Geometry check sheet. Reference: the model listing, model coordinates, mm. Round coordinates to 2 decimals unless told otherwise and drop trailing zeros. Loops run counter-clockwise (first coordinate to the right, second up) from the corner with the lowest first, then second, coordinate; pieces in that order, holes last. Notation, with made-up numbers: (4, -17) - (12, -17) arc R15 cw to (12, 4) - close; hole circle Ø2 at (-31, -34). An arc over 180 degrees is marked (long way). Write item = value, one per line.
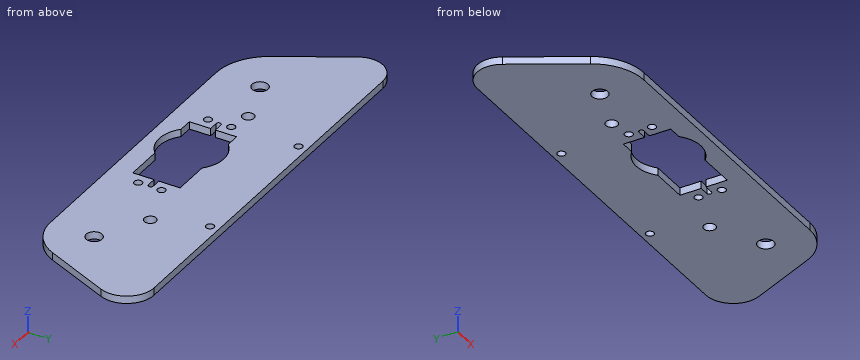
```python
from build123d import *

# Parameters (mm, degrees)
SKETCH1_R           = 3.429
SKETCH1_R_2         = 2.54
BOSS_EXTRUDE1_DEPTH = 3.2004
SKETCH2_R           = 1.7272
CUT_EXTRUDE1_DEPTH  = 3.2004
SKETCH5_R           = 1.7272
SKETCH5_W           = 40.894
SKETCH5_H           = 20.32
CUT_EXTRUDE3_DEPTH  = 4.2004
CUT_EXTRUDE4_DEPTH  = 3.2004
SKETCH9_R           = 13.885201093
CUT_EXTRUDE7_DEPTH  = 3.2004


with BuildPart() as part:
    # Sketch1 → Boss-Extrude1 (new body)
    with BuildSketch(Plane.XY):
        with BuildLine():
            Line((0, 0), (120.015, 0))
            ThreePointArc((120.015, 0), (130.351788397, 3.075697789), (137.325636158, 11.302152593))
            Line((137.325636158, 11.302152593), (149.69326877, 39.451329485))
            ThreePointArc((149.69326877, 39.451329485), (148.774539583, 50.600046625), (138.937102863, 55.925719911))
            Line((138.937102863, 55.925719911), (-26.54325766, 55.925719911))
            ThreePointArc((-26.54325766, 55.925719911), (-36.046025914, 50.429200208), (-36.019801229, 39.451329485))
            Line((-36.019801229, 39.451329485), (-19.648099871, 11.302152593))
            ThreePointArc((-19.648099871, 11.302152593), (-11.333429333, 3.027112684), (0, 0))
        make_face()
        with Locations((120.015, 18.90776)):
            Circle(SKETCH1_R, mode=Mode.SUBTRACT)
        with Locations((0, 18.90776)):
            Circle(SKETCH1_R, mode=Mode.SUBTRACT)
        with Locations((19.734727626, 25.566426992)):
            Circle(SKETCH1_R_2, mode=Mode.SUBTRACT)
        with Locations((99.400822531, 30.809360911)):
            Circle(SKETCH1_R_2, mode=Mode.SUBTRACT)
    extrude(amount=BOSS_EXTRUDE1_DEPTH)

    # Sketch2 → Cut-Extrude1 (cut)
    with BuildSketch(Plane(origin=(0, 0, 0), x_dir=(-1, 0, 0), z_dir=(0, 0, -1))):
        with Locations((-92.0115, 52.115719911)):
            Circle(SKETCH2_R)
        with Locations((-28.0035, 52.115719911)):
            Circle(SKETCH2_R)
    extrude(amount=-CUT_EXTRUDE1_DEPTH, mode=Mode.SUBTRACT)

    # Sketch5 → Cut-Extrude3 (cut, through all)
    with BuildSketch(Plane(origin=(0, 0, 0), x_dir=(-1, 0, 0), z_dir=(0, 0, -1))):
        with Locations((-79.746999972, 23.90776)):
            Circle(SKETCH5_R)
        with Locations((-29.246999972, 13.90776)):
            Circle(SKETCH5_R)
        with Locations((-29.246999972, 23.90776)):
            Circle(SKETCH5_R)
        with Locations((-79.746999972, 13.90776)):
            Circle(SKETCH5_R)
        with Locations((-54.496999972, 18.90776)):
            Rectangle(SKETCH5_W, SKETCH5_H)
    extrude(amount=-CUT_EXTRUDE3_DEPTH, mode=Mode.SUBTRACT)

    # Sketch6 → Cut-Extrude4 (cut)
    with BuildSketch(Plane.XY.offset(3.2004)):
        with BuildLine():
            Line((29.985999972, 19.92376), (34.049999972, 19.92376))
            Line((34.049999972, 19.92376), (34.049999972, 17.89176))
            Line((34.049999972, 17.89176), (29.985999972, 17.89176))
            ThreePointArc((29.985999972, 17.89176), (28.969999972, 18.90776), (29.985999972, 19.92376))
        make_face()
        with BuildLine():
            Line((74.943999972, 19.92376), (79.007999972, 19.92376))
            ThreePointArc((79.007999972, 19.92376), (80.023999972, 18.90776), (79.007999972, 17.89176))
            Line((79.007999972, 17.89176), (74.943999972, 17.89176))
            Line((74.943999972, 17.89176), (74.943999972, 19.92376))
        make_face()
    extrude(amount=-CUT_EXTRUDE4_DEPTH, mode=Mode.SUBTRACT)

    # Sketch9 → Cut-Extrude7 (cut)
    with BuildSketch(Plane(origin=(0, 0, 0), x_dir=(-1, 0, 0), z_dir=(0, 0, -1))):
        with Locations((-49.53, 18.90776)):
            Circle(SKETCH9_R)
    extrude(amount=-CUT_EXTRUDE7_DEPTH, mode=Mode.SUBTRACT)


solid = part.part
```
(1) Section check A-A (x = 36). Enter the section's corners in (y, z).
Answers follow:
outline = (0, 0) - (8.75, 0) - (8.75, 3.2) - (0, 3.2) - close; (29.07, 0) - (55.93, 0) - (55.93, 3.2) - (29.07, 3.2) - close
(2) Section check C-C (x = 56.5). Enter the section's corners in (y, z), then the cut area to 3 significant figures.
Answers follow:
outline = (0, 0) - (6.9, 0) - (6.9, 3.2) - (0, 3.2) - close; (30.92, 0) - (55.93, 0) - (55.93, 3.2) - (30.92, 3.2) - close
area = 102 mm²
(3) Scan lines: L1, parallel to Y at x = 0, z = 1.7; L2, parallel to Y at x = 68.5, z = 0.2; L3, parallel to X at y = 30, z = 2.75. Record each from-to range of solid material in increasing order. Write a range as [from, to].
Answers follow:
L1 = [0, 15.48], [22.34, 55.93]
L2 = [0, 8.75], [29.07, 55.93]
L3 = [-30.52, 41.18], [57.88, 96.99], [101.81, 145.54]
(4) Gauge pin test, flat ends, axial feed: pin 1 (1 mm diameter, centred on y = 26, z = 2, fed in from +X); pin 2 (1.6 mm diameter, centred on y = 15.5, z = 1, fed in from +X); pin 3 (1.5 mm diameter, centred on y = 6.5, z = 2, fed in from +X). Record the tip position at first contact, or that the pin passes through.
Answers follow:
pin_1 = 144
pin_2 = 139.52
pin_3 = 134.9
(5) Section check D-D (x = -17). Enter the section's corners in (y, z), then the cut area to 3 significant figures.
Answers follow:
outline = (7.64, 0) - (55.93, 0) - (55.93, 3.2) - (7.64, 3.2) - close
area = 155 mm²
(6) Section check B-B (z = 1.45). State how many separate pieces and enclosed holes the cut face has, then the cut area to 3 significant figures.
Answers follow:
separate_pieces = 1
enclosed_holes = 11
area = 8,400 mm²
